For this review, take the finished solid that the model builds, in its own axes (mm). Face numbers are marked on the shaded views. Round coordinates to 2 decimals unless told otherwise and drop trailing zeros. Loops run counter-clockwise (first coordinate to the right, second up) from the corner with the lowest first, then second, coordinate; pieces in that order, holes last. Notation, with made-up numbers: M -24.75,71.25 L -15.75,71.25 A24 ccw -15.75,90.25 Z; hole C -34.5,24.5 d3. An arc over 180 degrees is marked long. Write item = value, one per line. Start each with the question number.
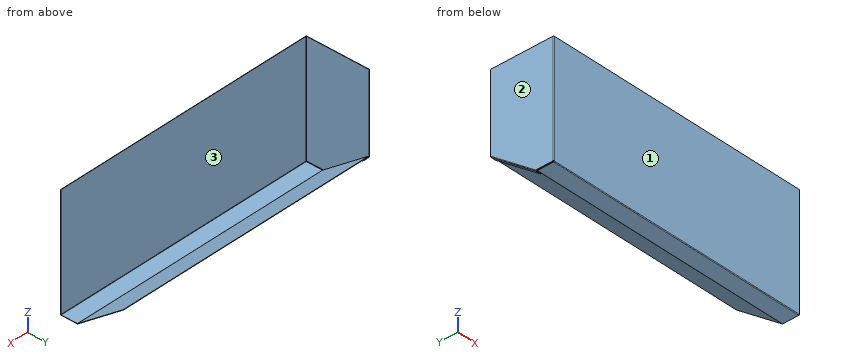
```python
from build123d import *

# Parameters (mm, degrees)
SKETCH2_W                    = 254
SKETCH2_H                    = 0.7366
BASE_FLANGE1_DEPTH           = 600
EDGE_FLANGE1_STRIP_W         = 4.4196
EDGE_FLANGE1_STRIP_H         = 0.7366
EDGE_FLANGE1_STRIP_CUT_DEPTH = 600
EDGE_FLANGE1_DEPTH           = 600
EDGE_FLANGE2_STRIP_CUT_DEPTH = 600
EDGE_FLANGE2_DEPTH           = 600
EDGE_FLANGE3_DEPTH           = 253.2634
CUT_EXTRUDE1_DEPTH           = 669.329179279
EDGE_FLANGE4_DEPTH           = 127.552071744


# Sheet-metal steps are written as plain solids
with BuildPart() as part:
    # Sketch2 → Base-Flange1 (new body)
    with BuildSketch(Plane(origin=(0, 0, 0), x_dir=(0, 0, -1), z_dir=(1, 0, 0))):
        with Locations((127, -0.3683)):
            Rectangle(SKETCH2_W, SKETCH2_H)
    extrude(amount=BASE_FLANGE1_DEPTH)

    # Edge-Flange1 strip (across the edge) → Edge-Flange1 strip cut (cut)
    with BuildSketch(Plane(origin=(600, 0, -254), x_dir=(0, 0, 1), z_dir=(-1, 0, 0))):
        with Locations((-1.4732, -0.3683)):
            Rectangle(EDGE_FLANGE1_STRIP_W, EDGE_FLANGE1_STRIP_H)
    extrude(amount=EDGE_FLANGE1_STRIP_CUT_DEPTH, mode=Mode.SUBTRACT)

    # Edge-Flange1 section (across the edge) → Edge-Flange1 (add)
    with BuildSketch(Plane(origin=(600, 0, -254), x_dir=(0, 0, 1), z_dir=(-1, 0, 0))):
        with BuildLine():
            Line((-0.7366, 0.7366), (-0.7366, 37.3634))
            Line((-0.7366, 37.3634), (0, 37.3634))
            Line((0, 37.3634), (0, 0.7366))
            ThreePointArc((0, 0.7366), (0.215745145, 0.215745145), (0.7366, 0))
            Line((0.7366, 0), (0.7366, -0.7366))
            ThreePointArc((0.7366, -0.7366), (-0.30510971, -0.30510971), (-0.7366, 0.7366))
        make_face()
    extrude(amount=EDGE_FLANGE1_DEPTH)

    # Edge-Flange2 strip (across the edge) → Edge-Flange2 strip cut (cut)
    with BuildSketch(Plane(origin=(600, 37.3634, -254), x_dir=(0, -0.6018150231520416, 0.7986355100472979), z_dir=(-1, 0, 0))):
        Polygon((-3.09973151, 2.88951852), (-0.439949833, -0.64013098), (0.148325083, -0.196834034), (-2.511456593, 3.332815466), align=None)
    extrude(amount=EDGE_FLANGE2_STRIP_CUT_DEPTH, mode=Mode.SUBTRACT)

    # Edge-Flange2 section (across the edge) → Edge-Flange2 (add)
    with BuildSketch(Plane(origin=(600, 37.3634, -254), x_dir=(0, -0.6018150231520416, 0.7986355100472979), z_dir=(-1, 0, 0))):
        with BuildLine():
            Line((-0.7366, 0.246462912), (-0.7366, 129.753537088))
            Line((-0.7366, 129.753537088), (0, 129.753537088))
            Line((0, 129.753537088), (0, 0.246462912))
            ThreePointArc((0, 0.246462912), (0.038064796, 0.012736302), (0.148325083, -0.196834034))
            Line((0.148325083, -0.196834034), (-0.439949833, -0.64013098))
            ThreePointArc((-0.439949833, -0.64013098), (-0.660470409, -0.220990307), (-0.7366, 0.246462912))
        make_face()
    extrude(amount=EDGE_FLANGE2_DEPTH)

    # Edge-Flange3 section (across the edge) → Edge-Flange3 (add)
    with BuildSketch(Plane(origin=(-0.7366, 0, -253.2634), x_dir=(1, 0, 0), z_dir=(0, 0, 1))):
        with BuildLine():
            Line((-0.7366, 0.7366), (-0.7366, 141.432479218))
            Line((-0.7366, 141.432479218), (0, 141.432479218))
            Line((0, 141.432479218), (0, 0.7366))
            ThreePointArc((0, 0.7366), (0.215745145, 0.215745145), (0.7366, 0))
            Line((0.7366, 0), (0.7366, -0.7366))
            ThreePointArc((0.7366, -0.7366), (-0.30510971, -0.30510971), (-0.7366, 0.7366))
        make_face()
    extrude(amount=EDGE_FLANGE3_DEPTH)

    # Sketch16 → Cut-Extrude1 (cut, through all)
    with BuildSketch(Plane.ZY.offset(1.4732)):
        Polygon((-254.439949833, 38.00353098), (-176.50064699, 141.432479218), (-254.439949833, 141.432479218), align=None)
    extrude(amount=-CUT_EXTRUDE1_DEPTH, mode=Mode.SUBTRACT)

    # Edge-Flange4 section (across the edge) → Edge-Flange4 (add)
    with BuildSketch(Plane(origin=(-0.7366, 40.00816229, -253.851674917), x_dir=(5.5927072616139335e-15, -0.6018150231520416, 0.7986355100472979), z_dir=(-2.7888745978675463e-15, 0.7986355100472979, 0.6018150231520416))):
        with BuildLine():
            Line((-0.7366, 0.7366), (-0.7366, 11.9634))
            Line((-0.7366, 11.9634), (0, 11.9634))
            Line((0, 11.9634), (0, 0.7366))
            ThreePointArc((0, 0.7366), (0.215745145, 0.215745145), (0.7366, 0))
            Line((0.7366, 0), (0.7366, -0.7366))
            ThreePointArc((0.7366, -0.7366), (-0.30510971, -0.30510971), (-0.7366, 0.7366))
        make_face()
    extrude(amount=EDGE_FLANGE4_DEPTH)


solid = part.part
```
(1) Add section B-B on z = -94. Write out the cut boundary in (x, y), and give its area (3 significant figures).
(2) Wall thickness on L1, parallel to Y at x = 502, z = -73; L2, parallel to X at y = 72, z = -169.5; L3, parallel to Z at x = 347, y = 7: over which ranges is each line inside the solid? List them lowest first.
(3) Add section A-A on x = 208. Write out the cut boundary in (y, z).
(4) For pin 1 Ø2 at (x, y) = (507.5, 68.5) entering from +Z; pin 2 Ø3 at (y, z) = (25.5, -99.5) entering from +X; pin 3 Ø4 at (x, y) = (163, 114.5) entering from +Z, all flat-tipped, find the tip position at first contact; note any pin that passes through.
(5) Draft analysis for pull direction Y (two halves, no side actions). For the marked faces 1, 2 and 3, state which applies: +Y half, -Y half, draft (parallel to the pull), parting line (faces both ways), or undercut.
Answer sheet:
q1.outline = M -1.47,0.74 A1.47 ccw 0,-0.74 L 600,-0.74 L 600,0 L 0,0 A0.74 cw -0.74,0.74 L -0.74,141.43 L -1.47,141.43 Z
q1.area = 547 mm²
q2.L1 = -0.74 to 0
q2.L2 = -1.47 to -0.74
q2.L3 = -254.74 to -254
q3.outline = M -0.74,-253.26 A1.47 ccw 0.74,-254.74 L 37.12,-254.74 A1.47 ccw 38,-254.44 L 141.43,-176.5 L 140.99,-175.91 L 37.56,-253.85 A0.74 cw 37.12,-254 L 0.74,-254 A0.74 cw 0,-253.26 L 0,0 L -0.74,0 Z
q4.pin_1 = -229.78
q4.pin_2 = -0.74
q4.pin_3 = -194.37
q5.face_1 = -Y half
q5.face_2 = draft
q5.face_3 = undercut
